```python
from build123d import *

# Parameters (mm, degrees)
F1_DEPTH = 660.4
F3_DEPTH = 38.101


with BuildPart() as f1:
    # F0 (on Front) → F1 (new body)
    with BuildSketch(Plane.XZ):
        Polygon((19.05, 15.875), (19.05, 19.05), (-19.05, 19.05), (-19.05, -19.05), (-15.875, -19.05), (-15.875, 15.875), align=None)
    extrude(amount=F1_DEPTH)

    # F2 (on face) → F3 (cut, through all)
    with BuildSketch(Plane.XY.offset(19.05)):
        Polygon((-19.05, -660.4), (19.05, -660.4), (-19.05, -622.3), align=None)
        Polygon((-19.05, -38.1), (19.05, 0), (-19.05, 0), align=None)
    extrude(amount=-F3_DEPTH, mode=Mode.SUBTRACT)


solid = f1.part
```
Part model, mm, in its own coordinate system. A direction names the side the tool comes from. Coordinates: 2 decimals unless noted, no trailing zeros. Order: outer loops, then holes, each group sorted by start corner. A loop starts at its lowest first (then second) coordinate and runs counter-clockwise, first axis right, second up. Notation, with made-up numbers: (18, 5.25) - (31, 5.25) arc R24 ccw to (31, 16.25) - close; hole circle Ø3 at (30, 24.5). An arc over 180 degrees is marked (long way). Return JSON: item names as keys, results as strings. Group by question number.
Item 1: Which spindle directions (+Z, -Z, +X, -X, +Y, -Y) get a long thin tool onto all of the face, cutting with end or side? Do faces 1 (the face through (-15.875, -326, -2)), 2 (the face through (-8.56, -27.61, 17.02)). Say none if no direction does.
Item 2: Drill centre lines: probe 1 along Z at (x, y) = (7.5, -75) (3 decimals); probe 2 along X at (y, z) = (-225, 11.5) (3 decimals); probe 3 along Y at (x, z) = (-3, 17). Where is each one in solid material? Low to high. Write a range as from..to.
Item 3: Pin check, flat tips, straight feed: pin 1 (12 mm diameter, centred on y = -140.5, z = -15, fed in from +X) (3 decimals); pin 2 (10 mm diameter, centred on x = 9.5, y = -124, fed in from -Z) (3 decimals). Stop position of each tip, or through.
Item 4: Cut at C-C (z = -6). List the corners of the cut face in (x, y) (3 decimals).
Item 5: Cut at B-B (y = -454.5). List the corners of the cut face in (x, z) (3 decimals), plus the area to 3 significant figures.
Item 6: Cut at A-A (x = -4.5). List the corners of the cut face in (y, z) (3 decimals).
Check values:
{
 "1": {"face 1": "-Z, +X, +Y, -Y", "face 2": "+Z, -Z, -X, +Y"},
 "2": {"probe 1": "z = 15.875..19.05", "probe 2": "x = -19.05..-15.875", "probe 3": "y = -638.35..-22.05"},
 "3": {"pin 1": "stops at x = -15.875", "pin 2": "stops at z = 15.875"},
 "4": {"outline": "(-19.05, -622.3) - (-15.875, -625.475) - (-15.875, -34.925) - (-19.05, -38.1) - close"},
 "5": {"outline": "(-19.05, -19.05) - (-15.875, -19.05) - (-15.875, 15.875) - (19.05, 15.875) - (19.05, 19.05) - (-19.05, 19.05) - close", "area": "232 mm2"},
 "6": {"outline": "(-636.85, 15.875) - (-23.55, 15.875) - (-23.55, 19.05) - (-636.85, 19.05) - close"}
}
